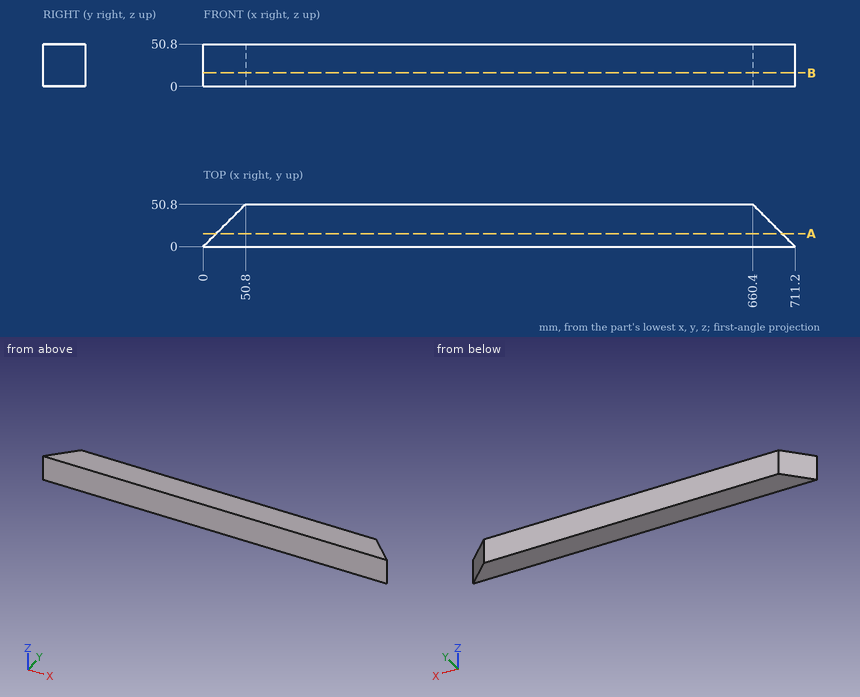
Drawing for the job (mm, zero at the part's lowest x, y, z). Give positions to 0.01 mm unless a question says otherwise; leave off trailing zeros. Order: outer loops, then holes, each group sorted by start corner. A loop starts at its lowest first (then second) coordinate and runs counter-clockwise, first axis right, second up. Notation, with made-up numbers: M -25.75,70 L 19.25,70 A11 cw 19.25,87 Z; hole C 7,55.25 d7. An arc over 180 degrees is marked long. Put each result on its own line as item: value. Start each with the question number.
(1) Drill centre lines: line 1 along X through (y, z) = (35, 48.5); line 2 along X through (y, z) = (20, 11.5); line 3 along Y through (x, z) = (39, 2.5). Where is each one in solid material? Low to high.
(2) Flat gauge pin, fed straight in: pin 1 Ø1 at (y, z) = (24, 44.5) entering from +X. Where does the tip first touch, or does it go through?
(3) Saw through at B-B, the plane z = 16. Write the cut outline in (x, y).
(4) Saw through at A-A, the plane y = 15.5. Write the cut outline in (x, z), then the cut area to 3 significant figures.
Check result:
1. line 1: x = 35 to 676.2
1. line 2: x = 20 to 691.2
1. line 3: y = 0 to 39
2. pin 1: stops at x = 687.7
3. outline: M 0,0 L 711.2,0 L 660.4,50.8 L 50.8,50.8 Z
4. outline: M 15.5,0 L 695.7,0 L 695.7,50.8 L 15.5,50.8 Z
4. area: 34,600 mm2
